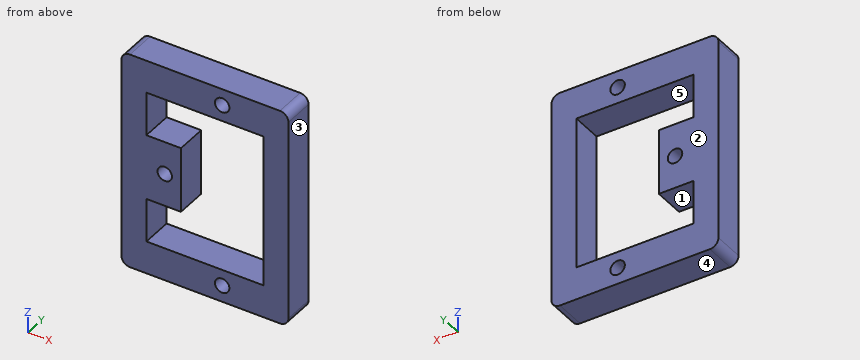
```python
from build123d import *

# Parameters (mm, degrees)
SKETCH1_W           = 24.9682
SKETCH1_H           = 32.639
BOSS_EXTRUDE1_DEPTH = 4.6482
SKETCH2_R           = 1.0795
CUT_EXTRUDE1_DEPTH  = 4.6482
FILLET1_R           = 1.27


with BuildPart() as part:
    # Sketch1 → Boss-Extrude1 (new body)
    with BuildSketch(Plane(origin=(0, 0, 0), x_dir=(1, 0, 0), z_dir=(0, 1, 0))):
        Rectangle(SKETCH1_W, SKETCH1_H)
        Polygon((8.743727626, 11.43), (8.743727626, -11.43), (-8.743727626, -11.43), (-8.743727626, -4.8895), (-3.575272374, -4.8895), (-3.575272374, 4.8895), (-8.743727626, 4.8895), (-8.743727626, 11.43), align=None, mode=Mode.SUBTRACT)
    extrude(amount=BOSS_EXTRUDE1_DEPTH)

    # Sketch2 → Cut-Extrude1 (cut)
    with BuildSketch(Plane(origin=(0, 4.6482, 0), x_dir=(1, 0, 0), z_dir=(0, 1, 0))):
        with Locations(Location((2.584227626, 13.85062, 0), (0, 0, 270))):
            Circle(SKETCH2_R)
        with Locations(Location((2.584227626, -13.85062, 0), (0, 0, 270))):
            Circle(SKETCH2_R)
        with Locations(Location((-6.000972374, 0, 0), (0, 0, 270))):
            Circle(SKETCH2_R)
    extrude(amount=-CUT_EXTRUDE1_DEPTH, mode=Mode.SUBTRACT)

    # Fillet1
    fillet1_edges = [part.edges().sort_by_distance(p)[0] for p in [
        (-12.4841, 2.3241, 16.3195),
        (12.4841, 2.3241, 16.3195),
        (12.4841, 2.3241, -16.3195),
        (-12.4841, 2.3241, -16.3195),
    ]]
    fillet(fillet1_edges, radius=FILLET1_R)


solid = part.part
```
Work out the finished part from the listing and answer in its coordinate system (mm). Face numbers are marked on the shaded views. A direction names the side the tool comes from. Give positions to 0.01 mm unless a question says otherwise; leave off trailing zeros. Loops run counter-clockwise (first coordinate to the right, second up) from the corner with the lowest first, then second, coordinate; pieces in that order, holes last. Notation, with made-up numbers: (80.25, 62.5) -> (96.25, 62.5) arc R32 cw to (96.25, 96.5) -> close; hole circle Ø1 at (0, -1). An arc over 180 degrees is marked (long way). Write item = value, one per line. Start each with the question number.
(1) Given pin 1 Ø10 at (x, z) = (5.5, -6) entering from +Y, flat-ended and moving along its own axis, determine where the tip first touches the part or whether it passes through.
(2) Which of the six approach directions +Z, -Z, +X, -X, +Y, -Y give full straight-line access (tool end or side, diameter ignored) to the marked faces 1 and 2?
(3) Find the intervals of material crossed by probe 1 along X at (y, z) = (1.7, 0); probe 2 along X at (y, z) = (4.15, 3); probe 3 along Z at (x, y) = (8.5, 4.3), in increasing order. Write a range as from..to.
(4) Find section D-D on y = 1.65. Give the vertices of the cut face in (x, z).
(5) The mould has two halves that part along Z. Classify the marked faces 3, 4 and 5: +Z half, -Z half, draft (parallel to the pull), parting line (faces both ways), or undercut.
(6) Find section B-B on x = 7.25. Give the vertices of the cut face in (y, z), and give its area (3 significant figures).
(7) Find section A-A on z = -8. Give the vertices of the cut face in (x, y).
(8) Find section C-C on z = 0. Give the vertices of the cut face in (x, y), and give its area (3 significant figures).
From the geometry:
q1.pin_1 = 4.65
q2.face_1 = +Y, -Y
q2.face_2 = +Z, -Z, +X, -X, +Y
q3.probe_1 = -12.48..-7.08, -4.92..-3.58, 8.74..12.48
q3.probe_2 = -12.48..-3.58, 8.74..12.48
q3.probe_3 = -16.32..-11.43, 11.43..16.32
q4.outline = (-12.48, -15.05) arc R1.27 ccw to (-11.21, -16.32) -> (11.21, -16.32) arc R1.27 ccw to (12.48, -15.05) -> (12.48, 15.05) arc R1.27 ccw to (11.21, 16.32) -> (-11.21, 16.32) arc R1.27 ccw to (-12.48, 15.05) -> close; hole (-8.74, -11.43) -> (8.74, -11.43) -> (8.74, 11.43) -> (-8.74, 11.43) -> (-8.74, 4.89) -> (-3.58, 4.89) -> (-3.58, -4.89) -> (-8.74, -4.89) -> close; hole circle Ø2.16 at (-6, 0); hole circle Ø2.16 at (2.58, -13.85); hole circle Ø2.16 at (2.58, 13.85)
q5.face_3 = draft
q5.face_4 = -Z half
q5.face_5 = undercut
q6.outline = (0, -16.32) -> (4.65, -16.32) -> (4.65, -11.43) -> (0, -11.43) -> close; (0, 11.43) -> (4.65, 11.43) -> (4.65, 16.32) -> (0, 16.32) -> close
q6.area = 45.5 mm^2
q7.outline = (-12.48, 0) -> (-8.74, 0) -> (-8.74, 4.65) -> (-12.48, 4.65) -> close; (8.74, 0) -> (12.48, 0) -> (12.48, 4.65) -> (8.74, 4.65) -> close
q8.outline = (-12.48, 0) -> (-7.08, 0) -> (-7.08, 4.65) -> (-12.48, 4.65) -> close; (-4.92, 0) -> (-3.58, 0) -> (-3.58, 4.65) -> (-4.92, 4.65) -> close; (8.74, 0) -> (12.48, 0) -> (12.48, 4.65) -> (8.74, 4.65) -> close
q8.area = 48.8 mm^2
